The listing builds one solid part. Answer for the finished solid, in the listing's coordinates (mm). Face numbers are marked on the shaded views. Give positions to 0.01 mm unless a question says otherwise; leave off trailing zeros. Write each loop counter-clockwise with the first axis right and the second up, starting at its lowest first coordinate (ties: lowest second). Pieces come first, ordered by that corner, then holes. Notation, with made-up numbers: M 73,15 L 77,15 A26 ccw 77,34 Z; hole C 9,58 d10. An arc over 180 degrees is marked long. Return JSON: item names as keys, results as strings.
from build123d import *

# Parameters (mm, degrees)
BOSS_EXTRUDE1_DEPTH                            = 4.7625
SKETCH5_R                                      = 10
CUT_EXTRUDE1_DEPTH                             = 81.819371269
CSK_FOR_M8_FLAT_HEAD_MACHINE_SCREW1_AT_2_COUNT = 2
CSK_FOR_M8_FLAT_HEAD_MACHINE_SCREW1_AT_2_PITCH = 25
FILLET1_R                                      = 25
M5_CLEARANCE_HOLE1_D                           = 5.5
M5_CLEARANCE_HOLE1_CSINK_D                     = 5.55
M5_CLEARANCE_HOLE1_CSINK_ANGLE                 = 90
FILLET2_R                                      = 5
CUT_EXTRUDE2_DEPTH                             = 81.819371269


with BuildPart() as part:
    # Sketch1 → Boss-Extrude1 (new body)
    with BuildSketch(Plane(origin=(0, 0, 0), x_dir=(1, 0, 0), z_dir=(0, 1, 0))):
        with BuildLine():
            Line((-12.5, -72.691742077), (12.5, -72.691742077))
            Line((12.5, -72.691742077), (12.5, -32.691742077))
            ThreePointArc((12.5, -32.691742077), (0, 35), (-12.5, -32.691742077))
            Line((-12.5, -32.691742077), (-12.5, -72.691742077))
        make_face()
    extrude(amount=BOSS_EXTRUDE1_DEPTH)

    # Sketch5 → Cut-Extrude1 (cut, through all)
    with BuildSketch(Plane.XZ):
        with Locations(Location((0, 0, 0), (0, 0, 270))):
            Circle(SKETCH5_R)
    extrude(amount=-CUT_EXTRUDE1_DEPTH, mode=Mode.SUBTRACT)

    # Sketch8 → CSK for M8 Flat Head Machine Screw1 (revolve, cut)
    with BuildSketch(Plane(origin=(0, 0, 37.691742077), x_dir=(0, 0, -1), z_dir=(1, 0, 0))):
        Polygon((0, 0), (0, 4.7625), (4.5, 4.7625), (4.5, 4.15), (8.65, 0), align=None)
    csk_for_m8_flat_head_machine_screw1 = revolve(axis=Axis((0, -6.35, 37.691742077), (0, 1, 0)), mode=Mode.SUBTRACT)

    # CSK for M8 Flat Head Machine Screw1 at 2: CSK for M8 Flat Head Machine Screw1 ×2
    with Locations(*[(0, 0, i * CSK_FOR_M8_FLAT_HEAD_MACHINE_SCREW1_AT_2_PITCH) for i in range(1, CSK_FOR_M8_FLAT_HEAD_MACHINE_SCREW1_AT_2_COUNT)]):
        add(csk_for_m8_flat_head_machine_screw1, mode=Mode.SUBTRACT)

    # Fillet1
    fillet1_edges = [part.edges().sort_by_distance(p)[0] for p in [
        (-12.5, 2.38125, 32.691742077),
        (12.5, 2.38125, 32.691742077),
    ]]
    fillet(fillet1_edges, radius=FILLET1_R)

    # M5 Clearance Hole1 (through all)
    with Locations(Plane(origin=(0, 0, 0), x_dir=(-1, 0, 0), z_dir=(0, -1, 0))):
        with Locations((10, 26), (24, 12), (24, -8), (-10, 26), (-24, 12), (-24, -8)):
            CounterSinkHole(M5_CLEARANCE_HOLE1_D / 2, M5_CLEARANCE_HOLE1_CSINK_D / 2, counter_sink_angle=M5_CLEARANCE_HOLE1_CSINK_ANGLE)

    # Fillet2
    fillet2_edges = [part.edges().sort_by_distance(p)[0] for p in [
        (12.5, 2.38125, 72.691742077),
        (-12.5, 2.38125, 72.691742077),
    ]]
    fillet(fillet2_edges, radius=FILLET2_R)

    # Sketch12 → Cut-Extrude2 (cut, through all)
    with BuildSketch(Plane(origin=(0, 4.7625, 0), x_dir=(1, 0, 0), z_dir=(0, 1, 0))):
        with BuildLine():
            Line((17, 3), (27, 3))
            ThreePointArc((27, 3), (30, 0), (27, -3))
            Line((27, -3), (17, -3))
            ThreePointArc((17, -3), (14, 0), (17, 3))
        make_face()
        with BuildLine():
            Line((14.142135624, -9.899494937), (21.213203436, -16.970562748))
            ThreePointArc((21.213203436, -16.970562748), (21.213203436, -21.213203436), (16.970562748, -21.213203436))
            Line((16.970562748, -21.213203436), (9.899494937, -14.142135624))
            ThreePointArc((9.899494937, -14.142135624), (9.899494937, -9.899494937), (14.142135624, -9.899494937))
        make_face()
        with BuildLine():
            Line((3, -17), (3, -27))
            ThreePointArc((3, -27), (0, -30), (-3, -27))
            Line((-3, -27), (-3, -17))
            ThreePointArc((-3, -17), (0, -14), (3, -17))
        make_face()
        with BuildLine():
            Line((-9.899494937, -14.142135624), (-16.970562748, -21.213203436))
            ThreePointArc((-16.970562748, -21.213203436), (-21.213203436, -21.213203436), (-21.213203436, -16.970562748))
            Line((-21.213203436, -16.970562748), (-14.142135624, -9.899494937))
            ThreePointArc((-14.142135624, -9.899494937), (-9.899494937, -9.899494937), (-9.899494937, -14.142135624))
        make_face()
        with BuildLine():
            Line((-17, -3), (-27, -3))
            ThreePointArc((-27, -3), (-30, 0), (-27, 3))
            Line((-27, 3), (-17, 3))
            ThreePointArc((-17, 3), (-14, 0), (-17, -3))
        make_face()
        with BuildLine():
            Line((-14.142135624, 9.899494937), (-21.213203436, 16.970562748))
            ThreePointArc((-21.213203436, 16.970562748), (-21.213203436, 21.213203436), (-16.970562748, 21.213203436))
            Line((-16.970562748, 21.213203436), (-9.899494937, 14.142135624))
            ThreePointArc((-9.899494937, 14.142135624), (-9.899494937, 9.899494937), (-14.142135624, 9.899494937))
        make_face()
        with BuildLine():
            Line((-3, 17), (-3, 27))
            ThreePointArc((-3, 27), (0, 30), (3, 27))
            Line((3, 27), (3, 17))
            ThreePointArc((3, 17), (0, 14), (-3, 17))
        make_face()
        with BuildLine():
            Line((9.899494937, 14.142135624), (16.970562748, 21.213203436))
            ThreePointArc((16.970562748, 21.213203436), (21.213203436, 21.213203436), (21.213203436, 16.970562748))
            Line((21.213203436, 16.970562748), (14.142135624, 9.899494937))
            ThreePointArc((14.142135624, 9.899494937), (9.899494937, 9.899494937), (9.899494937, 14.142135624))
        make_face()
    extrude(amount=-CUT_EXTRUDE2_DEPTH, mode=Mode.SUBTRACT)


solid = part.part
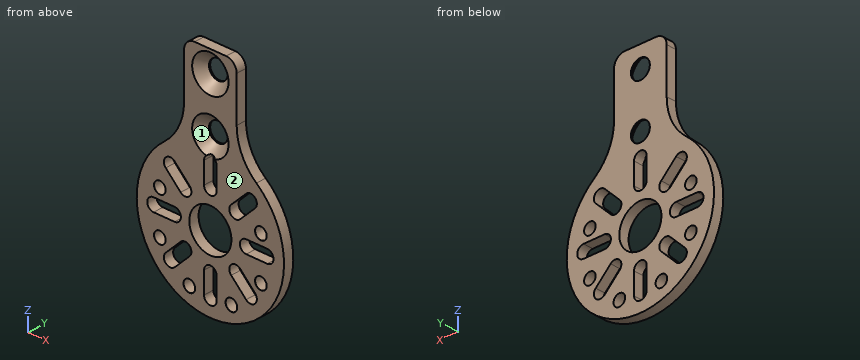
Item 1: A cutting plane is placed at B-B, the plane z = -12. Count the separate pieces of the cut face and the enclosed holes in it, plus the area to 3 significant figures.
Geometry results:
{"separate pieces": "5", "enclosed holes": "0", "area": "192 mm2"}
Item 2: A cutting plane is placed at A-A, the plane z = 0. Write down the section's boundary in (x, y), plus the area to 3 significant figures.
Geometry results:
{"outline": "M -35,0 L -30,0 L -30,4.76 L -35,4.76 Z; M -14,0 L -10,0 L -10,4.76 L -14,4.76 Z; M 10,0 L 14,0 L 14,4.76 L 10,4.76 Z; M 30,0 L 35,0 L 35,4.76 L 30,4.76 Z", "area": "85.7 mm2"}
Item 3: Given pin 1 Ø1.4 at (x, y) = (20, 1.5) entering from -Z; pin 2 Ø12 at (x, z) = (-26.5, 36.5) entering from -Y; pin 3 Ø1.4 at (y, z) = (3.5, 62.5) entering from +X; pin 4 Ø1.4 at (x, y) = (-22, 2.5) entering from -Z, each flat-ended and moving along its own axis, determine where each tip first touches the part or whether it passes through.
Geometry results:
{"pin 1": "stops at z = -29.2", "pin 2": "passes through", "pin 3": "stops at x = 12.5", "pin 4": "stops at z = -27.77"}
Item 4: A cutting plane is placed at D-D, the plane z = 25.5. Write down the section's boundary in (x, y), plus the area to 3 significant figures.
Geometry results:
{"outline": "M -23.97,0 L -3,0 L -3,4.76 L -23.97,4.76 Z; M 3,0 L 23.97,0 L 23.97,4.76 L 3,4.76 Z", "area": "200 mm2"}
Item 5: Find the intervals of material crossed by line 1 (Z direction, x = -5.5, y = 2.25); line 2 (Z direction, x = 8, y = 1); line 3 (X direction, y = 3.45, z = 12), in increasing order.
Geometry results:
{"line 1": "z = -34.57 to -8.35, 8.35 to 34.42, 40.96 to 59.42, 65.96 to 72.69", "line 2": "z = -34.07 to -27.89, -24.11 to -6, 6 to 72.67", "line 3": "x = -32.88 to -16.24, -9.02 to 9.02, 16.24 to 32.88"}
Item 6: Determine the mould class of the marked faces 1 and 2 for opening direction Z: +Z half, -Z half, draft (parallel to the pull), parting line (faces both ways), or undercut.
Geometry results:
{"face 1": "undercut", "face 2": "draft"}
